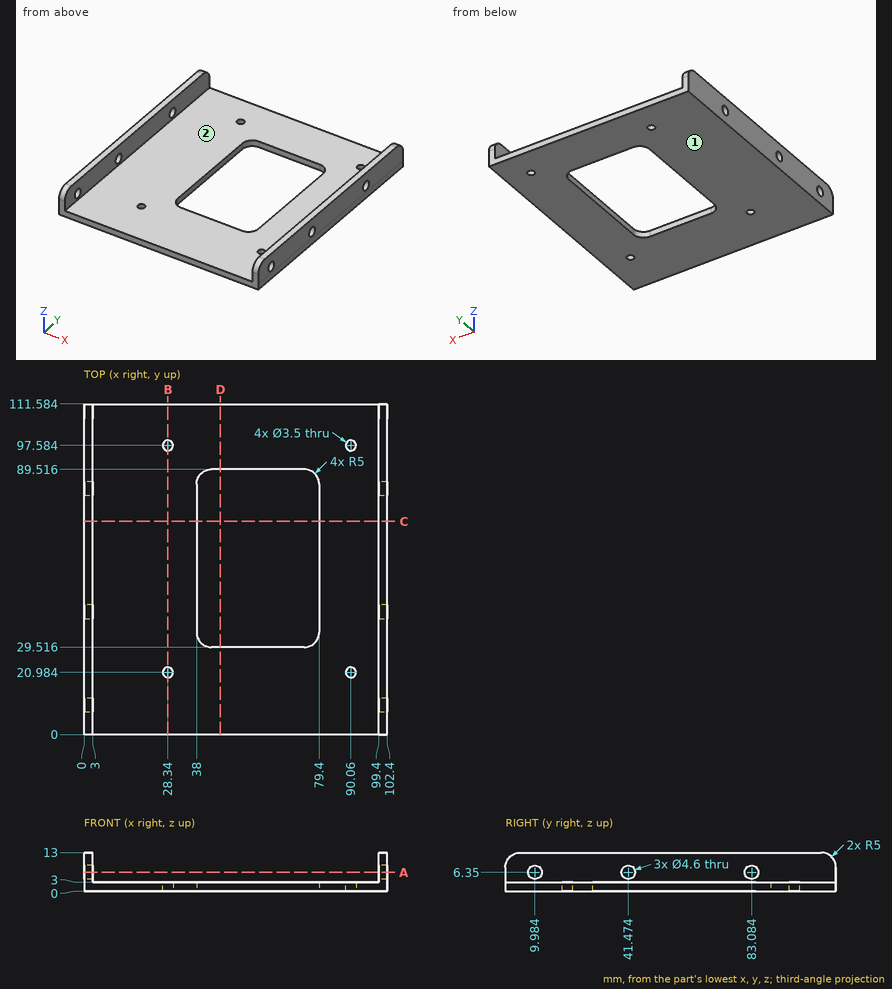
Drawing for the job (mm, zero at the part's lowest x, y, z). A direction names the side the tool comes from. Give positions to 0.01 mm unless a question says otherwise; leave off trailing zeros. Write each loop counter-clockwise with the first axis right and the second up, starting at its lowest first coordinate (ties: lowest second). Pieces come first, ordered by that corner, then holes. Notation, with made-up numbers: (35, 72.25) -> (50, 72.25) arc R21 ccw to (50, 87.25) -> close; hole circle Ø2 at (54, 12). An arc over 180 degrees is marked (long way). Put each result on its own line as item: value. Start each with the question number.
Item 1: Cut at C-C (y = 72). List the corners of the cut face in (x, z), then the cut area to 3 significant figures.
Item 2: Pin check, flat tips, straight feed: pin 1 Ø3 at (y, z) = (41.47, 6.35) entering from +X; pin 2 Ø5.5 at (x, y) = (28.34, 20.98) entering from +Z. Stop position of each tip, or through.
Item 3: Which spindle directions (+Z, -Z, +X, -X, +Y, -Y) get a long thin tool onto all of the face, cutting with end or side? Do the marked faces 1 and 2. Say none if no direction does.
Item 4: Cut at D-D (x = 46). List the corners of the cut face in (y, z), then the cut area to 3 significant figures.
Item 5: Wall check: L1, parallel to Y at x = 28.34, z = 1.65; L2, parallel to X at y = 106.5, z = 10.75; L3, parallel to X at y = 67, z = 1.75. Give the ranges that are in metal, low to high. Write a range as [from, to].
Item 6: Cut at B-B (x = 28.34). List the corners of the cut face in (y, z), then the cut area to 3 significant figures.
Item 7: Cut at A-A (z = 6.35). State how many separate pieces and enclosed holes the cut face has.
Answer list:
1. outline: (0, 0) -> (38, 0) -> (38, 3) -> (3, 3) -> (3, 13) -> (0, 13) -> close; (79.4, 0) -> (102.4, 0) -> (102.4, 13) -> (99.4, 13) -> (99.4, 3) -> (79.4, 3) -> close
1. area: 243 mm2
2. pin 1: passes through
2. pin 2: stops at z = 3
3. face 1: -Z, +X, -X, +Y, -Y
3. face 2: +Z, +Y, -Y
4. outline: (0, 0) -> (29.52, 0) -> (29.52, 3) -> (0, 3) -> close; (89.52, 0) -> (111.58, 0) -> (111.58, 3) -> (89.52, 3) -> close
4. area: 155 mm2
5. L1: y = [0, 19.23], [22.73, 95.83], [99.33, 111.58]
5. L2: x = [0, 3], [99.4, 102.4]
5. L3: x = [0, 38], [79.4, 102.4]
6. outline: (0, 0) -> (19.23, 0) -> (19.23, 3) -> (0, 3) -> close; (22.73, 0) -> (95.83, 0) -> (95.83, 3) -> (22.73, 3) -> close; (99.33, 0) -> (111.58, 0) -> (111.58, 3) -> (99.33, 3) -> close
6. area: 314 mm2
7. separate pieces: 8
7. enclosed holes: 0
